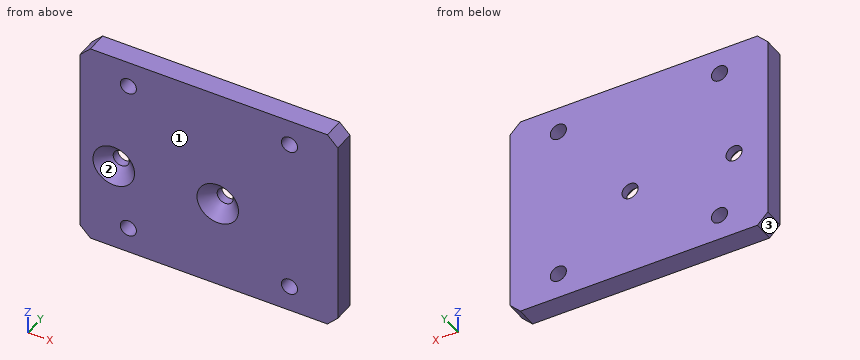
```python
from build123d import *

# Parameters (mm, degrees)
F1_DEPTH       = 4
F2_D           = 3.1
F3_D           = 3.1
F3_CSINK_D     = 8
F3_CSINK_ANGLE = 90
F4_W           = 49.6
F4_H           = 20
F5_DEPTH       = 4
F6_SIZE        = 2


with BuildPart() as f1:
    # F0 (on Front) → F1 (new body)
    with BuildSketch(Plane.XZ):
        Polygon((0, 24.9760837853), (0, 0), (49.6, 0), (49.6, 60), (0, 60), (0, 34.9760837853), align=None)
    extrude(amount=-F1_DEPTH)

    # F2 (through all)
    with Locations(Plane.XZ):
        with Locations((9.3, 55), (40.3, 55), (9.3, 25), (40.3, 25)):
            Hole(F2_D / 2)

    # F3 (through all)
    with Locations(Plane.XZ):
        with Locations((6.5, 37), (26.5, 37)):
            CounterSinkHole(F3_D / 2, F3_CSINK_D / 2, counter_sink_angle=F3_CSINK_ANGLE)

    # F4 (on face) → F5 (cut, through all)
    with BuildSketch(Plane.XZ):
        with Locations((24.8, 10)):
            Rectangle(F4_W, F4_H)
    extrude(amount=-F5_DEPTH, mode=Mode.SUBTRACT)

    # F6
    f6_edges = [f1.edges().sort_by_distance(p)[0] for p in [
        (49.6, 2, 60),
        (49.6, 2, 20),
        (0, 2, 60),
        (0, 2, 20),
    ]]
    chamfer(f6_edges, length=F6_SIZE)


solid = f1.part
```
Model file for the job. Use its own axes, mm. Face numbers are marked on the shaded views. Round coordinates to 2 decimals unless told otherwise and drop trailing zeros. Write each loop counter-clockwise with the first axis right and the second up, starting at its lowest first coordinate (ties: lowest second). Pieces come first, ordered by that corner, then holes. Notation, with made-up numbers: (46, -3.5) - (88, -3.5) arc R26 ccw to (88, 19.5) - close; hole circle Ø6 at (57.25, 51.5). An arc over 180 degrees is marked (long way). One line per item, written item: value.
(1) Cut at A-A, the plane x = 40.3. Give the cut face in (y, z).
Values follow:
outline: (0, 20) - (4, 20) - (4, 23.45) - (0, 23.45) - close; (0, 26.55) - (4, 26.55) - (4, 53.45) - (0, 53.45) - close; (0, 56.55) - (4, 56.55) - (4, 60) - (0, 60) - close
(2) Cut at C-C, the plane z = 55. Give the cut face in (x, y), plus the area to 3 significant figures.
Values follow:
outline: (0, 0) - (7.75, 0) - (7.75, 4) - (0, 4) - close; (10.85, 0) - (38.75, 0) - (38.75, 4) - (10.85, 4) - close; (41.85, 0) - (49.6, 0) - (49.6, 4) - (41.85, 4) - close
area: 174 mm²
(3) Drop flat-ended pins along their axis: P1, Ø4, axis at x = 6.5, z = 37, coming from the -Y side; P2, Ø3.5, axis at x = 26.5, z = 37, coming from the -Y side. Give the stop position or say it passes through.
Values follow:
P1: stops at y = 2
P2: stops at y = 2.25
(4) Two-plate mould, pull along Z, no slides. Class the marked faces 1, 2 and 3: pulls with the +Z half, pulls with the -Z half, needs draft (parallel to the pull), parting line crosses it, or undercut.
Values follow:
face 1: needs draft
face 2: undercut
face 3: pulls with the -Z half
(5) Cut at B-B, the plane y = 3. Give the cut face in (x, z).
Values follow:
outline: (0, 22) - (2, 20) - (47.6, 20) - (49.6, 22) - (49.6, 58) - (47.6, 60) - (2, 60) - (0, 58) - close; hole circle Ø3.1 at (6.5, 37); hole circle Ø3.1 at (9.3, 25); hole circle Ø3.1 at (9.3, 55); hole circle Ø3.1 at (26.5, 37); hole circle Ø3.1 at (40.3, 25); hole circle Ø3.1 at (40.3, 55)
(6) Cut at D-D, the plane x = 26.5. Give the cut face in (y, z), plus the area to 3 significant figures.
Values follow:
outline: (0, 20) - (4, 20) - (4, 35.45) - (2.45, 35.45) - (0, 33) - close; (0, 41) - (2.45, 38.55) - (4, 38.55) - (4, 60) - (0, 60) - close
area: 142 mm²
(7) Wall check: probe 1 along X at (y, z) = (3.25, 37); probe 2 along Z at (x, y) = (9.5, 3.55); probe 3 along Z at (x, y) = (9.3, 0.9). Give the ranges that are in metal, low to high.
Values follow:
probe 1: x = 0 to 4.95, 8.05 to 24.95, 28.05 to 49.6
probe 2: z = 20 to 23.46, 26.54 to 53.46, 56.54 to 60
probe 3: z = 20 to 23.45, 26.55 to 35.67, 38.33 to 53.45, 56.55 to 60
